CAD build for the part. Positions are in the model's coordinates, mm. A direction names the side the tool comes from. Give positions to 0.01 mm unless a question says otherwise; leave off trailing zeros. Loops run counter-clockwise (first coordinate to the right, second up) from the corner with the lowest first, then second, coordinate; pieces in that order, holes last. Notation, with made-up numbers: M -15,56.5 L 44,56.5 A29 ccw 44,76.5 Z; hole C -8.75,9 d11. An arc over 180 degrees is marked long. One line per question, with ' | ' between items.
```python
from build123d import *

# Parameters (mm, degrees)
SKETCH1_W           = 45
SKETCH1_H           = 20
BOSS_EXTRUDE1_DEPTH = 2
SKETCH2_R           = 8.826284226
BOSS_EXTRUDE3_DEPTH = 13
SKETCH2_5_R         = 8.826284226
BOSS_EXTRUDE4_DEPTH = 13


with BuildPart() as part:
    # Sketch1 → Boss-Extrude1 (new body)
    with BuildSketch(Plane.YZ):
        with Locations((22.5, 10)):
            Rectangle(SKETCH1_W, SKETCH1_H)
    extrude(amount=BOSS_EXTRUDE1_DEPTH)

    # Sketch2 → Boss-Extrude3 (add)
    with BuildSketch(Plane.YZ.offset(2)):
        with Locations(Location((10.096276732, 10, 0), (0, 0, 90))):
            Circle(SKETCH2_R)
    extrude(amount=BOSS_EXTRUDE3_DEPTH)

    # Sketch2_5 → Boss-Extrude4 (add)
    with BuildSketch(Plane.YZ.offset(2)):
        with Locations(Location((34.814683325, 10, 0), (0, 0, 90))):
            Circle(SKETCH2_5_R)
    extrude(amount=BOSS_EXTRUDE4_DEPTH)


solid = part.part
```
Item 1: Saw through at B-B on y = 22. Give the cut face in (x, z), and give its area (3 significant figures).
Conclusion:
outline: M 0,0 L 2,0 L 2,20 L 0,20 Z | area: 40.0 mm²
Item 2: Saw through at C-C on x = 5.75. Give the cut face in (y, z).
Conclusion:
outline: C 10.1,10 d17.65; C 34.81,10 d17.65
Item 3: 3-axis set-ups, long thin cutter, end or side, ignore diameter. For faces 1 (the flat face through (15, 10, 10)), 2 (the flat face through (2, 22, 10)): which of +Z, -Z, +X, -X, +Y, -Y reach the whole face in a straight line?
Conclusion:
face 1: +Z, -Z, +X, +Y, -Y | face 2: +X
Item 4: Mould opens along Y. For faces 3 (the cylindrical face through (8.41, 40.19, 3)), 4 (the flat face through (15, 35, 10)), 5 (the flat face through (1, 0, 10)), 6 (the flat face through (1, 45, 10)) say: pulls with the +Y half, pulls with the -Y half, needs draft (parallel to the pull), parting line crosses it, or undercut.
Conclusion:
face 3: undercut | face 4: needs draft | face 5: pulls with the -Y half | face 6: pulls with the +Y half
Item 5: Drill centre lines: line 1 along X through (y, z) = (7, 18.75); line 2 along Y through (x, z) = (13.5, 15.25); line 3 along Y through (x, z) = (10.75, 2.5). Where is each one in solid material? Low to high. Write a range as [from, to].
Conclusion:
line 1: [0, 2] | line 2: [3, 17.19], [27.72, 41.91] | line 3: [5.44, 14.75], [30.16, 39.47]
Item 6: Saw through at A-A on z = 10. Give the cut face in (x, y).
Conclusion:
outline: M 0,0 L 2,0 L 2,1.27 L 15,1.27 L 15,18.92 L 2,18.92 L 2,25.99 L 15,25.99 L 15,43.64 L 2,43.64 L 2,45 L 0,45 Z
Item 7: Saw through at D-D on z = 3.5. Give the cut face in (x, y), and give its area (3 significant figures).
Conclusion:
outline: M 0,0 L 2,0 L 2,4.13 L 15,4.13 L 15,16.07 L 2,16.07 L 2,28.84 L 15,28.84 L 15,40.79 L 2,40.79 L 2,45 L 0,45 Z | area: 400 mm²
Item 8: Drop flat-ended pins along their axis: P1, Ø6, axis at x = 13.5, y = 19.5, coming from the -Z side; P2, Ø1, axis at x = 5, z = 2.5, coming from the +Y side. Give the stop position or say it passes through.
Conclusion:
P1: z = 3.93 | P2: y = 40.19
